Check sheet for the modelled part. Datum: model origin and axes. Units: mm. Face numbers are marked on the shaded views. A direction names the side the tool comes from. Coordinates: 2 decimals unless noted, no trailing zeros. Loops run counter-clockwise (first coordinate to the right, second up) from the corner with the lowest first, then second, coordinate; pieces in that order, holes last. Notation, with made-up numbers: (84, -23) -> (134, -23) arc R38 ccw to (134, 15) -> close; hole circle Ø4 at (-24.75, -23.75). An arc over 180 degrees is marked (long way). Use one line per item in the form item = value.
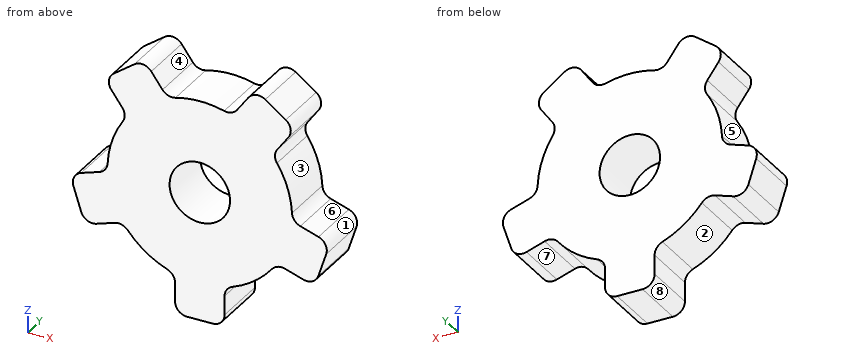
from build123d import *

# Parameters (mm, degrees)
SKETCH2_R           = 6.35
BOSS_EXTRUDE3_DEPTH = 11.684
FILLET1_R           = 2.54


with BuildPart() as part:
    # Sketch2 → Boss-Extrude3 (new body)
    with BuildSketch(Plane(origin=(0, 0, 0), x_dir=(1, 0, 0), z_dir=(0, 1, 0))):
        with BuildLine():
            Line((-5.207, 27.051), (5.207, 27.051))
            Line((5.207, 27.051), (5.207, 18.669))
            ThreePointArc((5.207, 18.669), (11.392188189, 15.680001858), (16.146222613, 10.721189548))
            Line((16.146222613, 10.721189548), (24.117978333, 13.311369995))
            Line((24.117978333, 13.311369995), (27.336081312, 3.407067434))
            Line((27.336081312, 3.407067434), (19.364325592, 0.816886988))
            ThreePointArc((19.364325592, 0.816886988), (18.432947696, -5.989227766), (15.185914365, -12.042940459))
            Line((15.185914365, -12.042940459), (20.112730349, -18.824120906))
            Line((20.112730349, -18.824120906), (11.68762737, -24.945316524))
            Line((11.68762737, -24.945316524), (6.760811385, -18.164136077))
            ThreePointArc((6.760811385, -18.164136077), (0, -19.381548184), (-6.760811385, -18.164136077))
            Line((-6.760811385, -18.164136077), (-11.68762737, -24.945316524))
            Line((-11.68762737, -24.945316524), (-20.112730349, -18.824120906))
            Line((-20.112730349, -18.824120906), (-15.185914365, -12.042940459))
            ThreePointArc((-15.185914365, -12.042940459), (-18.432947696, -5.989227766), (-19.364325592, 0.816886988))
            Line((-19.364325592, 0.816886988), (-27.336081312, 3.407067434))
            Line((-27.336081312, 3.407067434), (-24.117978333, 13.311369995))
            Line((-24.117978333, 13.311369995), (-16.146222613, 10.721189548))
            ThreePointArc((-16.146222613, 10.721189548), (-11.392188189, 15.680001858), (-5.207, 18.669))
            Line((-5.207, 18.669), (-5.207, 27.051))
        make_face()
        with Locations(Location((0, 0, 0), (0, 0, 270))):
            Circle(SKETCH2_R, mode=Mode.SUBTRACT)
    extrude(amount=BOSS_EXTRUDE3_DEPTH)

    # Fillet1
    fillet1_edges = [part.edges().sort_by_distance(p)[0] for p in [
        (-5.207, 5.842, -27.051),
        (5.207, 5.842, -27.051),
        (5.207, 5.842, -18.669),
        (16.146222613, 5.842, -10.721189548),
        (24.117978333, 5.842, -13.311369995),
        (27.336081312, 5.842, -3.407067434),
        (19.364325592, 5.842, -0.816886988),
        (15.185914365, 5.842, 12.042940459),
        (20.112730349, 5.842, 18.824120906),
        (11.68762737, 5.842, 24.945316524),
        (6.760811385, 5.842, 18.164136077),
        (-6.760811385, 5.842, 18.164136077),
        (-11.68762737, 5.842, 24.945316524),
        (-20.112730349, 5.842, 18.824120906),
        (-15.185914365, 5.842, 12.042940459),
        (-19.364325592, 5.842, -0.816886988),
        (-27.336081312, 5.842, -3.407067434),
        (-24.117978333, 5.842, -13.311369995),
        (-16.146222613, 5.842, -10.721189548),
        (-5.207, 5.842, -18.669),
    ]]
    fillet(fillet1_edges, radius=FILLET1_R)


solid = part.part
(1) Section check A-A, the plane x = 0. Record the boundary of the cut face in (y, z).
Established:
outline = (0, -27.05) -> (11.68, -27.05) -> (11.68, -6.35) -> (0, -6.35) -> close; (0, 6.35) -> (11.68, 6.35) -> (11.68, 19.38) -> (0, 19.38) -> close
(2) Mould release check, pull along Z, two halves, no side actions. Record for the marked faces 1, 2 and 3: +Z half, -Z half, draft (parallel to the pull), parting line (faces both ways), or undercut.
Established:
face_1 = parting line
face_2 = -Z half
face_3 = undercut
(3) Section check D-D, the plane x = -22.5. Record the boundary of the cut face in (y, z), plus the area to 3 significant figures.
Established:
outline = (0, -12.65) -> (11.68, -12.65) -> (11.68, -1.84) -> (0, -1.84) -> close
area = 126 mm²
(4) Section check B-B, the plane z = 0. Record the boundary of the cut face in (x, y).
Established:
outline = (-19.58, 0) -> (-6.35, 0) -> (-6.35, 11.68) -> (-19.58, 11.68) -> close; (6.35, 0) -> (19.58, 0) -> (19.58, 11.68) -> (6.35, 11.68) -> close
(5) Tool access check on the marked faces 4, 5, 6, 7 and 8. Record the directions out of +Z, -Z, +X, -X, +Y, -Y that give a thin tool (end or side, any length) a straight path to the whole face; none if there is none.
Established:
face_4 = +Z, +Y, -Y
face_5 = -X, +Y, -Y
face_6 = +Z, +X, +Y, -Y
face_7 = -Z, +Y, -Y
face_8 = -Z, -X, +Y, -Y
(6) Go/stop test with flat-tipped pins: P1, Ø2, axis at y = 2.5, z = -16.5, coming from the -X side; P2, Ø1, axis at y = 10.5, z = -15, coming from the -X side; P3, Ø2, axis at y = 4, z = -23, coming from the +X side. Record where each tip stops, or that it passes through.
Established:
P1 = -11.64
P2 = -12.86
P3 = 5.21
(7) Scan lines: line 1 along X through (y, z) = (6, -22.5); line 2 along Z through (x, y) = (18, 6); line 3 along X through (y, z) = (6.5, 4). Record each from-to range of solid material in increasing order.
Established:
line_1 = -5.21 to 5.21
line_2 = -11.32 to 7.19, 15.92 to 20.36
line_3 = -18.96 to -4.93, 4.93 to 18.96
(8) Section check C-C, the plane z = -22. Record the boundary of the cut face in (x, y).
Established:
outline = (-5.21, 0) -> (5.21, 0) -> (5.21, 11.68) -> (-5.21, 11.68) -> close
